Source: CAD feature listing. Evaluate the final solid. Frame: model axes, mm. Give positions to 0.01 mm unless a question says otherwise; leave off trailing zeros. Order: outer loops, then holes, each group sorted by start corner. A loop starts at its lowest first (then second) coordinate and runs counter-clockwise, first axis right, second up. Notation, with made-up numbers: (13, 71.5) -> (37, 71.5) arc R16 cw to (37, 75.5) -> close; hole circle Ø5 at (66, 60). An arc over 180 degrees is marked (long way). Answer in a Markdown table with one row per item.
```python
from build123d import *

# Parameters (mm, degrees)
SKETCH_1_W          = 52
SKETCH_1_H          = 46
EXTRUDE_1_DEPTH     = 3
SKETCH_2_R          = 10
SKETCH_2_R_2        = 1.6
CUT_EXTRUDE_1_DEPTH = 4


with BuildPart() as part:
    # 草图1 → 凸台-拉伸1 (new body)
    with BuildSketch(Plane.XY):
        Rectangle(SKETCH_1_W, SKETCH_1_H)
    extrude(amount=EXTRUDE_1_DEPTH)

    # 草图2 → 切除-拉伸1 (cut, through all)
    with BuildSketch(Plane.XY.offset(3)):
        Circle(SKETCH_2_R)
        with Locations((0, 15)):
            Circle(SKETCH_2_R_2)
        with Locations((12.990381057, -7.5)):
            Circle(SKETCH_2_R_2)
        with Locations((-12.990381057, -7.5)):
            Circle(SKETCH_2_R_2)
    extrude(amount=-CUT_EXTRUDE_1_DEPTH, mode=Mode.SUBTRACT)


solid = part.part
```
(1) Ray query, probe 1 along Y at (x, z) = (0, 1.3); probe 2 along X at (y, z) = (-7, 1.15); probe 3 along X at (y, z) = (8.5, 1.6). Return the intervals inside material, ascending.
A:
| item | result |
|---|---|
| probe 1 | y = -23 to -10, 10 to 13.4, 16.6 to 23 |
| probe 2 | x = -26 to -14.51, -11.47 to -7.14, 7.14 to 11.47, 14.51 to 26 |
| probe 3 | x = -26 to -5.27, 5.27 to 26 |
(2) Section query B-B (y = 6). Return the cut outline in (x, z).
A:
| item | result |
|---|---|
| outline | (-26, 0) -> (-8, 0) -> (-8, 3) -> (-26, 3) -> close; (8, 0) -> (26, 0) -> (26, 3) -> (8, 3) -> close |
(3) Pull-direction query (Y, two-part tool) for faces 1 (the flat face through (26, 0, 1)), 2 (the cylindrical face through (14.47, -8.11, 1.52)), 3 (the flat face through (0, 23, 1)); classes: +Y half, -Y half, draft (parallel to the pull), parting line (faces both ways), or undercut.
A:
| item | result |
|---|---|
| face 1 | draft |
| face 2 | undercut |
| face 3 | +Y half |
(4) Section query A-A (x = 0). Return the cut outline in (y, z), plus the area to 3 significant figures.
A:
| item | result |
|---|---|
| outline | (-23, 0) -> (-10, 0) -> (-10, 3) -> (-23, 3) -> close; (10, 0) -> (13.4, 0) -> (13.4, 3) -> (10, 3) -> close; (16.6, 0) -> (23, 0) -> (23, 3) -> (16.6, 3) -> close |
| area | 68.4 mm^2 |
(5) First-contact query: pin 1 Ø3 at (x, y) = (0, 15) entering from -Z. Flat tip, straight axial feed; report the tip coordinate or a pass-through.
A:
| item | result |
|---|---|
| pin 1 | passes through |
(6) Section query C-C (z = 1). Return the cut outline in (x, y).
A:
| item | result |
|---|---|
| outline | (-26, -23) -> (26, -23) -> (26, 23) -> (-26, 23) -> close; hole circle Ø3.2 at (-12.99, -7.5); hole circle Ø20 at (0, 0); hole circle Ø3.2 at (0, 15); hole circle Ø3.2 at (12.99, -7.5) |
(7) Section query D-D (x = 12). Return the cut outline in (y, z).
A:
| item | result |
|---|---|
| outline | (-23, 0) -> (-8.76, 0) -> (-8.76, 3) -> (-23, 3) -> close; (-6.24, 0) -> (23, 0) -> (23, 3) -> (-6.24, 3) -> close |
